Autodesk Fusion 360 part; units mm, degrees
sketch "Sketch3" plane through (0, 0, 0) normal (0, 0, 1) x (1, 0, 0)
  line L0 (0, 0) -> (76.5, 0)
  line L1 (76.5, 0) -> (76.5, 3)
  line L2 (76.5, 3) -> (0, 3)
  line L3 (0, 3) -> (0, 0)
  line L4 (0, 75) -> (76.5, 75)
  line L5 (76.5, 75) -> (76.5, 77.9078)
  line L6 (76.5, 77.9078) -> (0, 77.9078)
  line L7 (0, 77.9078) -> (0, 75)
  dimension "d24" = 76.5
  dimension "d25" = 3
  dimension "d26" = 76.5
  dimension "d27" = 72
extrude "Extrude4" add sketch "Sketch3" along normal blind 20 makes body 1 at (51, 3, 13.3333) makes body 2 at (51, 77.9078, 13.3333)
sketch "Sketch4" plane through (0, 0, 20) normal (0, 0, 1) x (-1, 0, 0)
  line L0 (0, -3) -> (0, 0)
  line L1 (0, 0) -> (-76.5, 0)
  line L2 (-76.5, 0) -> (-76.5, -3)
  line L3 (-76.5, -3) -> (0, -3)
  line L4 (0, -77.9078) -> (0, -75)
  line L5 (0, -75) -> (-76.5, -75)
  line L6 (-76.5, -75) -> (-76.5, -77.9078)
  line L7 (-76.5, -77.9078) -> (0, -77.9078)
  line L8 (0, -77.9078) -> (-76.5, -77.9078)
  line L9 (-76.5, -77.9078) -> (-76.5, 0)
  line L10 (-76.5, 0) -> (0, 0)
  line L11 (0, 0) -> (0, -77.9078)
extrude "Extrude5" add sketch "Sketch4" along normal blind 3 bodies 1 2
sketch "Sketch5" plane through (0, 0, 23) normal (0, 0, 1) x (-1, 0, 0)
  line L0 (0, 0) -> (-76.5, 0)
  line L1 (-76.5, 0) -> (-76.5, -77.9078)
  line L2 (-76.5, -77.9078) -> (0, -77.9078)
  line L3 (0, -77.9078) -> (0, 0)
  line L4 (0, -77.9078) -> (-76.5, 0) construction
  line L5 (-73.5, -64.7039) -> (-3, -64.7039)
  line L6 (-3, -64.7039) -> (-3, -13.2039)
  line L7 (-3, -13.2039) -> (-73.5, -13.2039)
  line L8 (-73.5, -13.2039) -> (-73.5, -64.7039)
  line L9 (-73.5, -64.7039) -> (-3, -13.2039) construction
  line L10 (-3, -64.7039) -> (-73.5, -13.2039) construction
  line L11 (-4, -14.2039) -> (-72.5, -14.2039)
  line L12 (-72.5, -14.2039) -> (-72.5, -63.7039)
  line L13 (-72.5, -63.7039) -> (-4, -63.7039)
  line L14 (-4, -63.7039) -> (-4, -14.2039)
  line L15 (0, -10.2039) -> (-76.5, -10.2039)
  line L16 (-76.5, -10.2039) -> (-76.5, -67.7039)
  line L17 (-76.5, -67.7039) -> (0, -67.7039)
  line L18 (0, -67.7039) -> (0, -10.2039)
  point P0 (-38.25, -38.9539)
  dimension "d35" = 70.5
  dimension "d36" = 51.5
  dimension "d38" = 3
extrude "Extrude8" add sketch "Sketch5" along normal blind 7.25 contours L1 L3 L15 L16 L17 L18 bodies 1
extrude "Extrude9" add sketch "Sketch5" along normal blind 6 contours L5 L6 L7 L8 bodies 1
extrude "Extrude6" [suppressed]
extrude "Extrude7" [suppressed]
equation "board_width = 51 mm"
equation "board_length = 70 mm"
equation "tolerance = 0.25 mm"
equation "board_holder_depth = 6 mm"
equation "board_thickness = 1.25 mm"
equation "board_overhang = 1 mm"
equation "thickness = 3 mm"
equation "bottom_part_gap = 72 mm"
equation "bottom_part_height = 20 mm"
equation "d24 = board_length + thickness * 2 + tolerance * 2"
equation "d25 = thickness"
equation "d26 = board_length + thickness * 2 + tolerance * 2"
equation "d27 = bottom_part_gap"
equation "d28 = bottom_part_height"
equation "d30 = thickness"
equation "d33 = board_holder_depth + board_thickness"
equation "d35 = board_length + tolerance * 2"
equation "d36 = board_width + tolerance * 2"
equation "d38 = thickness"
equation "d39 = board_holder_depth"
equation "d41 = board_holder_depth + board_thickness"
equation "d43 = board_holder_depth"
Input: part model. Units: mm. Frame: model coordinates. A direction names the side the tool comes from. Coordinates: 2 decimals unless noted, no trailing zeros. Loops run counter-clockwise (first coordinate to the right, second up) from the corner with the lowest first, then second, coordinate; pieces in that order, holes last.
Q1. Section C-C, the plane z = 2.5. Return the cut outline in (x, y), and give its area (3 significant figures).
Results are:
outline: (0, 0) - (76.5, 0) - (76.5, 3) - (0, 3) - close; (0, 75) - (76.5, 75) - (76.5, 77.91) - (0, 77.91) - close
area: 452 mm2
Q2. Section D-D, the plane x = 14.5. Return the cut outline in (y, z), and give its area (3 significant figures).
Results are:
outline: (0, 0) - (3, 0) - (3, 20) - (75, 20) - (75, 0) - (77.91, 0) - (77.91, 23) - (67.7, 23) - (67.7, 30.25) - (64.7, 30.25) - (64.7, 29) - (63.7, 29) - (63.7, 23) - (14.2, 23) - (14.2, 29) - (13.2, 29) - (13.2, 30.25) - (10.2, 30.25) - (10.2, 23) - (0, 23) - close
area: 407 mm2
Q3. Mould query, pull axis X, two halves, no side actions, for faces 1 (the flat face through (38, 2, 0)), 2 (the flat face through (72.5, 39, 26)), 3 (the flat face through (0, 39, 24)), 4 (the flat face through (76.5, 39, 24)). Classes: +X half, -X half, draft (parallel to the pull), parting line (faces both ways), or undercut.
Results are:
face 1: draft
face 2: undercut
face 3: -X half
face 4: +X half
Q4. Section A-A, the plane z = 26.5. Return the cut outline in (x, y).
Results are:
outline: (0, 10.2) - (76.5, 10.2) - (76.5, 67.7) - (0, 67.7) - close; hole (4, 14.2) - (72.5, 14.2) - (72.5, 63.7) - (4, 63.7) - close
Q5. Contact query for flat-ended pins moving along their axis: pin 1 (3 mm diameter, centred on x = 31, z = 26, fed in from -Y); pin 2 (5 mm diameter, centred on x = 23, y = 65.5, fed in from -Z); pin 3 (5 mm diameter, centred on x = 19, y = 73.5, fed in from +Z). Output: stop coordinate, or through.
Results are:
pin 1: stops at y = 10.2
pin 2: stops at z = 20
pin 3: stops at z = 23
Q6. Set-up query: faces 5 (the flat face through (39, 38, 20)), 6 (the flat face through (39, 63.704, 26)), 7 (the flat face through (39, 67.704, 27)), 8 (the flat face through (38, 10.204, 27)). Return all of +Z, -Z, +X, -X, +Y, -Y with unobstructed straight access to the full face (end or side cutting, diameter ignored); none if empty.
Results are:
face 5: -Z, +X, -X
face 6: +Z
face 7: +Z, +X, -X, +Y
face 8: +Z, +X, -X, -Y
Q7. Section B-B, the plane y = 60.5. Return the cut outline in (x, z).
Results are:
outline: (0, 20) - (76.5, 20) - (76.5, 30.25) - (73.5, 30.25) - (73.5, 29) - (72.5, 29) - (72.5, 23) - (4, 23) - (4, 29) - (3, 29) - (3, 30.25) - (0, 30.25) - close
Q8. Line query: line 1 along Y through (x, z) = (53, 28.5); line 2 along Y through (x, z) = (67, 15); line 3 along X through (y, z) = (52.5, 23.5). Output: solid intervals per line, ascending.
Results are:
line 1: y = 10.2 to 14.2, 63.7 to 67.7
line 2: y = 0 to 3, 75 to 77.91
line 3: x = 0 to 4, 72.5 to 76.5
